```python
from build123d import *

# Parameters (mm, degrees)
SKETCH_1_W           = 22
SKETCH_1_H           = 12
EXTRUDE_1_DEPTH      = 9
FILLET_1_R           = 2
SKETCH_2_R           = 4
CUT_EXTRUDE_1_DEPTH  = 8
SKETCH_3_R           = 5
CUT_EXTRUDE_2_DEPTH  = 1
EXTRUDE_2_DEPTH      = 6
CUT_EXTRUDE_5_DEPTH  = 3
SKETCH_8_R           = 2.5
CUT_EXTRUDE_6_DEPTH  = 6
SKETCH_11_R          = 2
CUT_EXTRUDE_9_DEPTH  = 23.135943621
SKETCH_12_W          = 27.17111841
SKETCH_12_H          = 33.234136994
CUT_EXTRUDE_10_DEPTH = 10


with BuildPart() as part:
    # Эскиз1 → Бобышка-Вытянуть1 (new body)
    with BuildSketch(Plane(origin=(0, 0, 0), x_dir=(1, 0, 0), z_dir=(0, 1, 0))):
        Rectangle(SKETCH_1_W, SKETCH_1_H)
    extrude(amount=EXTRUDE_1_DEPTH)

    # Скругление1
    fillet_1_edges = [part.edges().sort_by_distance(p)[0] for p in [
        (11, 4.5, 6),
        (-11, 4.5, 6),
        (-11, 4.5, -6),
        (11, 4.5, -6),
    ]]
    fillet(fillet_1_edges, radius=FILLET_1_R)

    # Эскиз2 → Вырез-Вытянуть1 (cut)
    with BuildSketch(Plane(origin=(0, 0, 0), x_dir=(1, 0, 0), z_dir=(0, 1, 0))):
        with Locations(Location((0, 0, 0), (0, 0, 270))):
            Circle(SKETCH_2_R)
    extrude(amount=CUT_EXTRUDE_1_DEPTH, mode=Mode.SUBTRACT)

    # Эскиз3 → Вырез-Вытянуть2 (cut)
    with BuildSketch(Plane.XZ.offset(-8)):
        with Locations(Location((0, 0, 0), (0, 0, 270))):
            Circle(SKETCH_3_R)
    extrude(amount=-CUT_EXTRUDE_2_DEPTH, mode=Mode.SUBTRACT)

    # Эскиз6 → Бобышка-Вытянуть2 (add)
    with BuildSketch(Plane(origin=(0, 9, 0), x_dir=(1, 0, 0), z_dir=(0, 1, 0))):
        Polygon((6.92820323, 0), (3.464101615, 6), (-3.464101615, 6), (-6.92820323, 0), (-3.464101615, -6), (3.464101615, -6), align=None)
    extrude(amount=EXTRUDE_2_DEPTH)

    # Эскиз7 → Вырез-Вытянуть5 (cut)
    with BuildSketch(Plane(origin=(0, 9, 0), x_dir=(1, 0, 0), z_dir=(0, 1, 0))):
        Polygon((5.773502692, 0), (2.886751346, 5), (-2.886751346, 5), (-5.773502692, 0), (-2.886751346, -5), (2.886751346, -5), align=None)
    extrude(amount=CUT_EXTRUDE_5_DEPTH, mode=Mode.SUBTRACT)

    # Эскиз8 → Вырез-Вытянуть6 (cut)
    with BuildSketch(Plane(origin=(0, 9, 0), x_dir=(1, 0, 0), z_dir=(0, 1, 0))):
        with Locations(Location((0, 0, 0), (0, 0, 90))):
            Circle(SKETCH_8_R)
    extrude(amount=CUT_EXTRUDE_6_DEPTH, mode=Mode.SUBTRACT)

    # Эскиз11 → Вырез-Вытянуть9 (cut, through all)
    with BuildSketch(Plane(origin=(0, 0, -6), x_dir=(-1, 0, 0), z_dir=(0, 0, -1))):
        with Locations((7, 4.5)):
            Circle(SKETCH_11_R)
    cut_extrude_9 = extrude(amount=-CUT_EXTRUDE_9_DEPTH, mode=Mode.SUBTRACT)

    # Зеркальное отражение6: Вырез-Вытянуть9 across plane
    add(cut_extrude_9.mirror(Plane(origin=(0, 0, 0), x_dir=(0, 0, 1), z_dir=(1, 0, 0))), mode=Mode.SUBTRACT)

    # Эскиз12 → Вырез-Вытянуть10 (cut)
    with BuildSketch(Plane.XY):
        Rectangle(SKETCH_12_W, SKETCH_12_H)
    extrude(amount=-CUT_EXTRUDE_10_DEPTH, mode=Mode.SUBTRACT)


solid = part.part
```
Geometry: final body of the model. Coordinates: model frame, mm. A direction names the side the tool comes from. Coordinates: 2 decimals unless noted, no trailing zeros. Order: outer loops, then holes, each group sorted by start corner. A loop starts at its lowest first (then second) coordinate and runs counter-clockwise, first axis right, second up. Notation, with made-up numbers: (38.5, -40) -> (85.5, -40) arc R32 cw to (85.5, -9) -> close; hole circle Ø5 at (11, 16). An arc over 180 degrees is marked (long way). Write each question's results on one line, items separated by ' | '. Start each with the question number.
1) Cut plane D-D, the plane z = 3.75. Output: boundary loops of the cut face in (x, y).
2) Set-up query: faces 1 (the flat face through (-8, 9, 3)), 2 (the flat face through (5.172, 11.958, 3.042)), 3 (the cylindrical face through (5.002, 4.588, 2.958)), 4 (the cylindrical face through (0, 4, 4)), 5 (the flat face through (2.6, 9, 4.5)). Return all of +Z, -Z, +X, -X, +Y, -Y with unobstructed straight access to the full face (end or side cutting, diameter ignored); none if empty.
3) Material intervals for line 1 along Y through (x, z) = (-7, 1.8); line 2 along X through (y, z) = (3.5, 3.25); line 3 along X through (y, z) = (3.75, 2.25), sorted ascending.
4) Cut plane B-B, the plane y = 2.25. Output: boundary loops of the cut face in (x, z), and give its area (3 significant figures).
5) Mould query, pull axis X, two halves, no side actions, for faces 6 (the cylindrical face through (-5.002, 4.588, 2.958)), 7 (the flat face through (-11, 4, 2)), 8 (the flat face through (-7, 8, 0)). Classes: released by +X, released by -X, zero draft, split by the parting line, or undercut.
6) First-contact query: pin 1 (2.5 mm diameter, centred on x = 7, y = 4.5, fed in from -Z); pin 2 (1.5 mm diameter, centred on y = 12, z = 3, fed in from -X); pin 3 (1.5 mm diameter, centred on x = 0.5, y = 10.5, fed in from -Z); pin 4 (1.5 mm diameter, centred on x = -8.5, z = 3.5, fed in from +Y). Flat tips, straight axial feed; report the tip coordinate or a pass-through.
7) Cut plane C-C, the plane x = 8.75. Output: boundary loops of the cut face in (y, z), and give its area (3 significant figures).
8) Cut plane A-A, the plane z = 1. Output: boundary loops of the cut face in (x, y), and give its area (3 significant figures).
Checks:
1) outline: (-11, 0) -> (-1.39, 0) -> (-1.39, 8) -> (-3.31, 8) -> (-3.31, 9) -> (-3.61, 9) -> (-3.61, 12) -> (3.61, 12) -> (3.61, 9) -> (3.31, 9) -> (3.31, 8) -> (1.39, 8) -> (1.39, 0) -> (11, 0) -> (11, 9) -> (4.76, 9) -> (4.76, 15) -> (-4.76, 15) -> (-4.76, 9) -> (-11, 9) -> close; hole circle Ø4 at (-7, 4.5); hole circle Ø4 at (7, 4.5)
2) face 1: +Z, -X, +Y | face 2: +Z, +X, +Y | face 3: +Z, -Z | face 4: -Z, -Y | face 5: -Z
3) line 1: 0 to 2.5, 6.5 to 9 | line 2: -11 to -8.73, -5.27 to -2.33, 2.33 to 5.27, 8.73 to 11 | line 3: -11 to -8.85, -5.15 to -3.31, 3.31 to 5.15, 8.85 to 11
4) outline: (-11, 0) -> (-4, 0) arc R4 cw to (4, 0) -> (11, 0) -> (11, 4) arc R2 ccw to (9, 6) -> (-9, 6) arc R2 ccw to (-11, 4) -> close | area: 105 mm^2
5) face 6: undercut | face 7: released by -X | face 8: zero draft
6) pin 1: through | pin 2: x = -5.63 | pin 3: z = 5 | pin 4: y = 9
7) outline: (0, 0) -> (3.53, 0) -> (3.53, 6) -> (0, 6) -> close; (5.47, 0) -> (9, 0) -> (9, 6) -> (5.47, 6) -> close | area: 42.4 mm^2
8) outline: (-11, 0) -> (-3.87, 0) -> (-3.87, 8) -> (-4.9, 8) -> (-4.9, 9) -> (-5.2, 9) -> (-5.2, 12) -> (-2.29, 12) -> (-2.29, 15) -> (-6.35, 15) -> (-6.35, 9) -> (-11, 9) -> close; (2.29, 12) -> (5.2, 12) -> (5.2, 9) -> (4.9, 9) -> (4.9, 8) -> (3.87, 8) -> (3.87, 0) -> (11, 0) -> (11, 9) -> (6.35, 9) -> (6.35, 15) -> (2.29, 15) -> close; hole circle Ø4 at (-7, 4.5); hole circle Ø4 at (7, 4.5) | area: 132 mm^2
